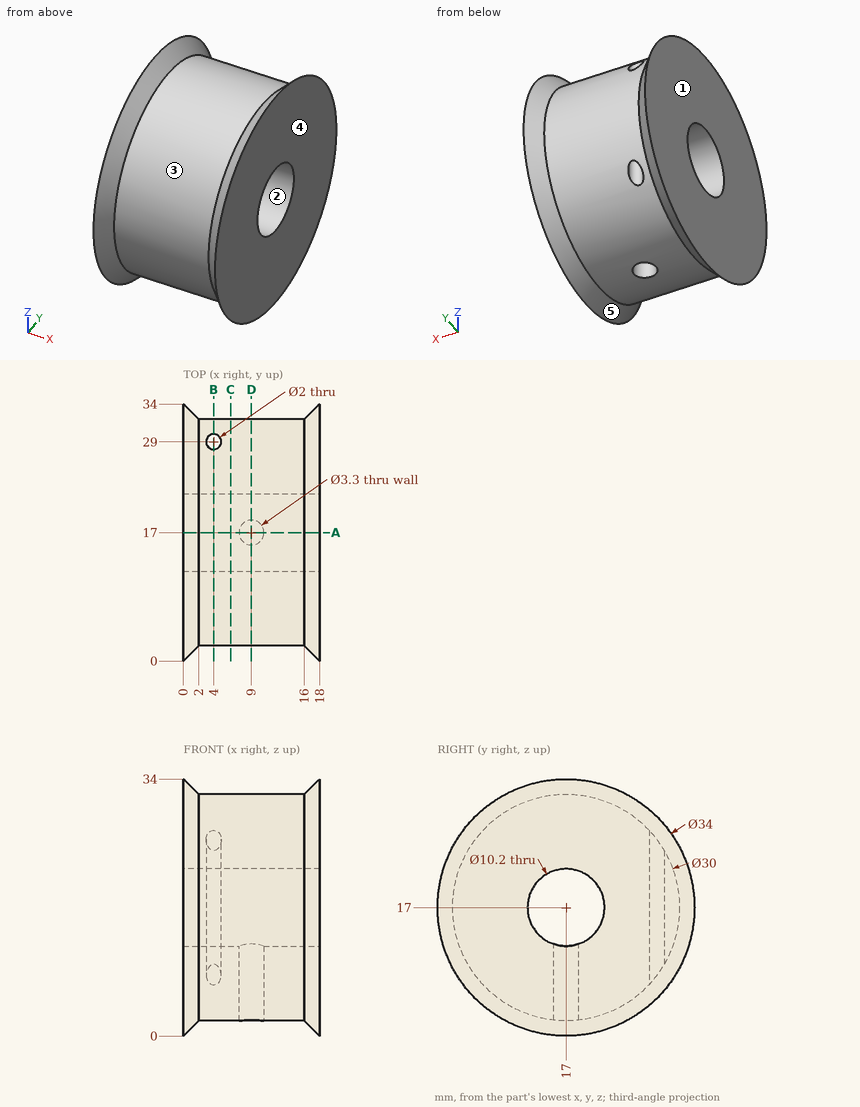
Can you work these out from the drawing? Everything is in mm from the part's minimum corner. A direction names the side the tool comes from. Coordinates: 2 decimals unless noted, no trailing zeros. Order: outer loops, then holes, each group sorted by start corner. A loop starts at its lowest first (then second) coordinate and runs counter-clockwise, first axis right, second up. Notation, with made-up numbers: M -13.5,15 L 21.5,15 A18 cw 21.5,21 Z; hole C 3,14 d1. An arc over 180 degrees is marked long. Answer as CSV lines item,"result". Start each with the question number.
1. I want a section at C-C, the plane x = 6.25. Write out the boundary of the cut face in (y, z).
2. On a 3-axis mill with a long thin cutter (end or side, diameter ignored), from which of +Z, -Z, +X, -X, +Y, -Y can I reach the whole of each face in a straight line? I mean the marked faces 4 and 5. Say none if no direction works.
3. I want a section at A-A, the plane y = 17. Write out the boundary of the cut face in (x, z), and give its area (3 significant figures).
4. We'd pull the mould along Z, two halves only. Please class the marked faces 1, 2 and 3: released by +Z, released by -Z, zero draft, split by the parting line, or undercut.
5. I want a section at B-B, the plane x = 4. Write out the boundary of the cut face in (y, z), and give its area (3 significant figures).
6. For pin 1 (2 mm diameter, centred on x = 3, z = 19, fed in from +Y); pin 2 (2.5 mm diameter, centred on x = 9, y = 17, fed in from -Z); pin 3 (6 mm diameter, centred on x = 5.5, z = 7.5, fed in from -Y), each with a flat end and sliding along its axis, tell me the tip position at first contact or that it passes through.
7. I need wall thicknesses on line 1 (Y direction, x = 4, z = 20.25); line 2 (Z direction, x = 5.75, y = 17); line 3 (X direction, y = 29, z = 18.25). Which ranges of each line are inside material? Lowest first, please. Write a range as [from, to].
8. I want a section at D-D, the plane x = 9. Write out the boundary of the cut face in (y, z).
Recorded:
1,outline,"C 17,17 d30; hole C 17,17 d10.2"
2,face 4,"+Z, -Z, +X, +Y, -Y"
2,face 5,"none"
3,outline,"M 0,0 L 2,2 L 7.35,2 L 7.35,11.9 L 0,11.9 Z; M 0,22.1 L 18,22.1 L 18,34 L 16,32 L 2,32 L 0,34 Z; M 10.65,2 L 16,2 L 18,0 L 18,11.9 L 10.65,11.9 Z"
3,area,"332 mm2"
4,face 1,"zero draft"
4,face 2,"undercut"
4,face 3,"split by the parting line"
5,outline,"M 28,6.8 L 28,27.2 A15 ccw long Z; M 30,9.52 A15 ccw 30,24.48 Z; hole C 17,17 d10.2"
5,area,"589 mm2"
6,pin 1,"stops at y = 31.97"
6,pin 2,"stops at z = 21.94"
6,pin 3,"stops at y = 3.48"
7,line 1,"y = [2.36, 13.07], [20.93, 28], [30, 31.64]"
7,line 2,"z = [2, 11.9], [22.1, 32]"
7,line 3,"x = [0, 3], [5, 18]"
8,outline,"M 15.35,2.09 L 15.35,12.17 A5.1 cw long 18.65,12.17 L 18.65,2.09 A15 ccw long Z"
